from build123d import *

# Parameters (mm, degrees)
F1_DEPTH = 3
F2_W     = 3
F2_H     = 6
F3_DEPTH = 3.001
F4_W     = 30
F4_H     = 3
F5_DEPTH = 3.001
F6_W     = 3
F6_H     = 20
F7_DEPTH = 3.001
F9_DEPTH = 3


with BuildPart() as f1:
    # F0 (on Right) → F1 (new body)
    with BuildSketch(Plane.YZ):
        Polygon((200, 116.077641), (0, 13), (0, 0), (20, 0), (20, 3), (180, 3), (180, 0), (200, 0), (200, 13), align=None)
    extrude(amount=F1_DEPTH)

    # F2 (on Right) → F3 (cut, through all)
    with BuildSketch(Plane.YZ):
        with Locations((1.5, 8)):
            Rectangle(F2_W, F2_H)
    extrude(amount=F3_DEPTH, mode=Mode.SUBTRACT)

    # F4 (on face) → F5 (cut, through all)
    with BuildSketch(Plane.YZ.offset(3)):
        Polygon((115, 3), (115, 4.5), (115, 6), (85, 6), (85, 3), align=None)
        Polygon((180, 6), (150, 6), (150, 4.5), (150, 3), (180, 3), align=None)
        with Locations((35, 4.5)):
            Rectangle(F4_W, F4_H)
    extrude(amount=-F5_DEPTH, mode=Mode.SUBTRACT)

    # F6 (on face) → F7 (cut, through all)
    with BuildSketch(Plane.YZ.offset(3)):
        with Locations((198.5, 84.531476)):
            Rectangle(F6_W, F6_H)
        with Locations((198.5, 36)):
            Rectangle(F6_W, F6_H)
    extrude(amount=-F7_DEPTH, mode=Mode.SUBTRACT)

    # F8 (on face) → F9 (join, through all)
    with BuildSketch(Plane.YZ.offset(3)):
        Polygon((23.070076, 28.265045), (24.444444, 25.598378), (51.111111, 39.342064), (49.736743, 42.00873), align=None)
        Polygon((147.51452, 92.402244), (148.888889, 89.735577), (175.555556, 103.479262), (174.181187, 106.145929), align=None)
        Polygon((85.292298, 60.333644), (86.666667, 57.666978), (113.333333, 71.410663), (111.958965, 74.07733), align=None)
    extrude(amount=-F9_DEPTH)


solid = f1.part
Input: part model. Units: mm. Frame: model coordinates. A direction names the side the tool comes from. Coordinates: 2 decimals unless noted, no trailing zeros. Write each loop counter-clockwise with the first axis right and the second up, starting at its lowest first coordinate (ties: lowest second). Pieces come first, ordered by that corner, then holes. Notation, with made-up numbers: M 26.5,-38.5 L 30.5,-38.5 A17 ccw 30.5,-31.5 Z; hole C -25.75,24 d11. An arc over 180 degrees is marked long. Answer as a JSON object with one key per item and string values. Group by question number.
(1) Set-up query: faces 1 (the face through (1.479, 187.949, 109.867)), 2 (the face through (0, 121, 46)). Return all of +Z, -Z, +X, -X, +Y, -Y with unobstructed straight access to the full face (end or side cutting, diameter ignored); none if empty.
(2) Section B-B on y = 162. Output: boundary loops of the cut face in (x, z), plus the area to 3 significant figures.
(3) Ray query, line 1 along Z through (x, y) = (1.6, 44.5); line 2 along Y through (x, z) = (2.4, 6.5); line 3 along Y through (x, z) = (0.2, 105). Return the intervals inside material, ascending. Write a range as [from, to].
(4) Contact query for flat-ended pins moving along their axis: P1, Ø1.5, axis at x = 1, y = 1.5, coming from the +Z side; P2, Ø8, axis at y = 154.5, z = 54, coming from the -X side; P3, Ø1, axis at x = 1.5, y = 86.5, coming from the +Z side; P4, Ø0.9, axis at x = 2, z = 88.5, coming from the +Y side. Output: stop coordinate, or through.
(5) Section C-C on y = 135. Output: boundary loops of the cut face in (x, z).
Result set:
{
 "1": {"face 1": "+Z, +X, -X", "face 2": "+Z, -Z, -X, +Y, -Y"},
 "2": {"outline": "M 0,6 L 3,6 L 3,99.87 L 0,99.87 Z", "area": "282 mm2"},
 "3": {"line 1": "z = [6, 39.31]", "line 2": "y = [3, 200]", "line 3": "y = [171.96, 174.77], [178.51, 200]"},
 "4": {"P1": "stops at z = 14.16", "P2": "stops at x = 0", "P3": "stops at z = 61.21", "P4": "stops at y = 197"},
 "5": {"outline": "M 0,3 L 3,3 L 3,82.58 L 0,82.58 Z"}
}
